from build123d import *

# Parameters (mm, degrees)
F0_W     = 50
F0_H     = 47
F1_DEPTH = 17.5
F2_R     = 20.5
F3_DEPTH = 45
F4_R     = 18.5
F5_DEPTH = 56.5
F6_R     = 6
F7_DEPTH = 25


with BuildPart() as f1:
    # F0 (on Top) → F1 (new body)
    with BuildSketch(Plane.XY):
        with Locations((25, 23.5)):
            Rectangle(F0_W, F0_H)
    extrude(amount=F1_DEPTH)

    # F2 (on face) → F3 (join)
    with BuildSketch(Plane.XY.offset(17.5)):
        with Locations((25, 23)):
            Circle(F2_R)
    extrude(amount=F3_DEPTH)

    # F4 (on face) → F5 (cut)
    with BuildSketch(Plane(origin=(0, 0, 0), x_dir=(1, 0, 0), z_dir=(0, 0, -1))):
        with Locations((25, -23)):
            Circle(F4_R)
    extrude(amount=-F5_DEPTH, mode=Mode.SUBTRACT)

    # F6 (on face) → F7 (cut)
    with BuildSketch(Plane.XY.offset(62.5)):
        with Locations((25, 35)):
            Circle(F6_R)
    extrude(amount=-F7_DEPTH, mode=Mode.SUBTRACT)


solid = f1.part
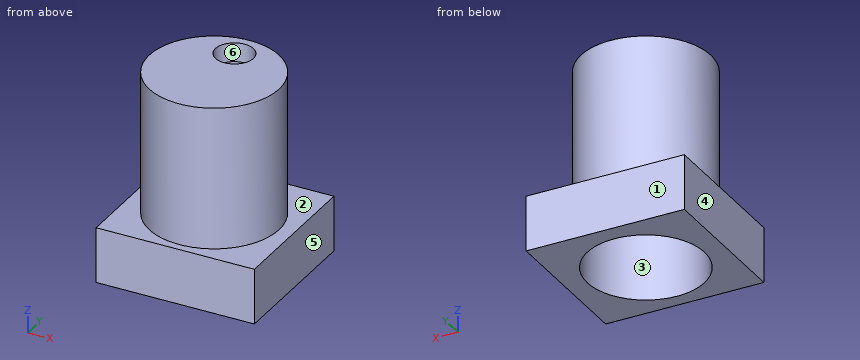
Could you check a few things on this model? Use its own coordinates, in mm. Face numbers are marked on the shaded views. A direction names the side the tool comes from. Give positions to 0.01 mm unless a question says otherwise; leave off trailing zeros. Write each loop counter-clockwise with the first axis right and the second up, starting at its lowest first coordinate (ties: lowest second). Pieces come first, ordered by that corner, then holes. Notation, with made-up numbers: (46, -20) - (85, -20) arc R12 cw to (85, -11) - close; hole circle Ø1 at (-5.5, 81.25). An arc over 180 degrees is marked (long way). Use CSV: the item, a comma, the result in double quotes. Start each with the question number.
Item 1: I want a section at B-B, the plane y = 37. Please give me the cut outline in (x, z).
Item 2: I'm going to push flat-ended pins straight in: pin 1 (1 mm diameter, centred on x = 34.5, y = 9.5, fed in from -Z); pin 2 (8 mm diameter, centred on x = 22.5, z = 25, fed in from -Y); pin 3 (2 mm diameter, centred on x = 39.5, z = 52, fed in from +Y). Where does each tip first touch, or does it pass through?
Item 3: If I drill on line 1 along Y through (x, z) = (25, 24.5); line 2 along Y through (x, z) = (25, 61.3); line 3 along X through (y, z) = (23, 15.5), over which ranges is the centre line in solid material (lowest first)?
Item 4: For the marked faces 1, 2 and 3, which set-ups out of +Z, -Z, +X, -X, +Y, -Y let a thin tool reach every point of the face, with its end or its side?
Item 5: If we mould it in two halves opening along X, with no side actions, what happens to the marked faces 4, 5 and 6? For each: pulls with the +X half, pulls with the -X half, needs draft (parallel to the pull), parting line crosses it, or undercut.
Item 6: I want a section at C-C, the plane y = 23. Please give me the cut outline in (x, z).
Item 7: I want a section at A-A, the plane x = 25. Please give me the cut outline in (y, z).
Item 8: I want a section at D-D, the plane z = 25.5. Please give me the cut outline in (x, y).
Findings:
1,outline,"(0, 0) - (12.91, 0) - (12.91, 56.5) - (19.34, 56.5) - (19.34, 62.5) - (10.03, 62.5) - (10.03, 17.5) - (0, 17.5) - close; (30.66, 56.5) - (37.09, 56.5) - (37.09, 0) - (50, 0) - (50, 17.5) - (39.97, 17.5) - (39.97, 62.5) - (30.66, 62.5) - close"
2,pin 1,"stops at z = 56.5"
2,pin 2,"stops at y = 2.5"
2,pin 3,"stops at y = 38.43"
3,line 1,"y = 2.5 to 4.5, 41.5 to 43.5"
3,line 2,"y = 2.5 to 29, 41 to 43.5"
3,line 3,"x = 0 to 6.5, 43.5 to 50"
4,face 1,"+Z, -Z, +X, -X, +Y"
4,face 2,"+Z"
4,face 3,"-Z"
5,face 4,"pulls with the -X half"
5,face 5,"pulls with the +X half"
5,face 6,"undercut"
6,outline,"(0, 0) - (6.5, 0) - (6.5, 56.5) - (43.5, 56.5) - (43.5, 0) - (50, 0) - (50, 17.5) - (45.5, 17.5) - (45.5, 62.5) - (4.5, 62.5) - (4.5, 17.5) - (0, 17.5) - close"
7,outline,"(0, 0) - (4.5, 0) - (4.5, 56.5) - (29, 56.5) - (29, 62.5) - (2.5, 62.5) - (2.5, 17.5) - (0, 17.5) - close; (41, 56.5) - (41.5, 56.5) - (41.5, 0) - (47, 0) - (47, 17.5) - (43.5, 17.5) - (43.5, 62.5) - (41, 62.5) - close"
8,outline,"circle Ø41 at (25, 23); hole circle Ø37 at (25, 23)"
